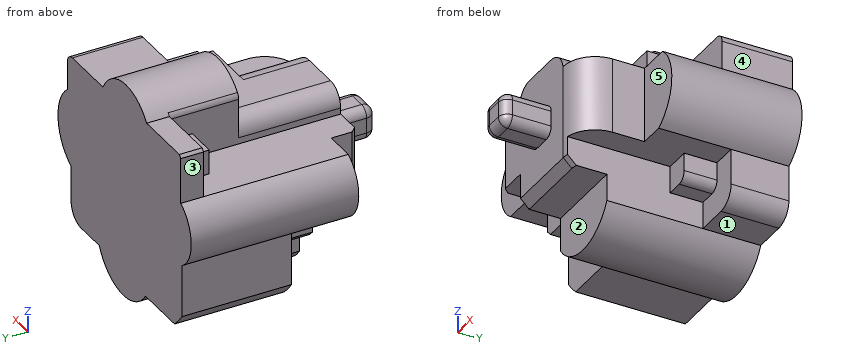
```python
from build123d import *

# Parameters (mm, degrees)
F0_W         = 19.224062562
F0_H         = 18.6825376004
F1_DEPTH     = 134.874
F2_DEPTH     = 108.204
F0_W_2       = 18.3131638914
F0_H_2       = 18.7943680212
F3_DEPTH     = 83.058
F0_W_3       = 17.1565823257
F0_H_3       = 13.6970020831
F4_DEPTH     = 25.4
F0_W_4       = 17.9688669741
F0_H_4       = 10.4478634894
F5_DEPTH     = 71.374
F0_W_5       = 14.1782090068
F0_H_5       = 15.0508098304
F6_DEPTH     = 50.546
F7_DEPTH     = 72.644
F8_DEPTH     = 85.852
F9_DEPTH     = 51.308
F10_DEPTH    = 93.472
F11_DEPTH    = 61.214
F12_DEPTH    = 32.258
F13_DEPTH    = 39.37
F14_DEPTH    = 12.7
F15_R        = 5.08
F16_R        = 10.16
F17_R        = 5.08
F18_T1_DEPTH = 68.0767879487
F19_R        = 10.16
F20_SIZE     = 3.0226
F21_R        = 17.78
F22_SIZE     = 4.8203104
F23_R        = 5.08
F24_R        = 5.08
F25_R        = 5.08
F26_R        = 5.08
F27_R        = 5.08


# Not quite as in the source:
# - a fillet or chamfer that OpenCascade refuses, or shapes differently, is made with other operations: its cross-section is extruded or revolved along the edge and cut away or added


with BuildPart() as f1:
    # F0 (on Front) → F1 (new body)
    with BuildSketch(Plane.XZ):
        Rectangle(F0_W, F0_H)
    extrude(amount=F1_DEPTH)

    # F0 (on Front) → F2 (join)
    with BuildSketch(Plane.XZ):
        Polygon((-21.2547723204, -33.8216274977), (25.389727205, -33.8216274977), (25.389727205, -18.7708176672), (39.5679362118, -18.7708176672), (39.5679362118, 23.3737640083), (21.5990692377, 23.3737640083), (21.5990692377, 33.8216274977), (-22.4113538861, 33.8216274977), (-22.4113538861, 20.1246254146), (-39.5679362118, 20.1246254146), (-39.5679362118, -15.0272594765), (-21.2547723204, -15.0272594765), align=None)
        Rectangle(F0_W, F0_H, mode=Mode.SUBTRACT)
    extrude(amount=F2_DEPTH)

    # F0 (on Front) → F3 (join)
    with BuildSketch(Plane.XZ):
        with Locations((-30.4113542661, -24.4244434871)):
            Rectangle(F0_W_2, F0_H_2)
    extrude(amount=F3_DEPTH)

    # F0 (on Front) → F4 (join)
    with BuildSketch(Plane.XZ):
        with Locations((-30.989645049, 26.9731264561)):
            Rectangle(F0_W_3, F0_H_3)
    extrude(amount=F4_DEPTH)

    # F0 (on Front) → F5 (join)
    with BuildSketch(Plane.XZ):
        with Locations((30.5835027248, 28.597695753)):
            Rectangle(F0_W_4, F0_H_4)
    extrude(amount=F5_DEPTH)

    # F0 (on Front) → F6 (join)
    with BuildSketch(Plane.XZ):
        with Locations((32.4788317084, -26.2962225825)):
            Rectangle(F0_W_5, F0_H_5)
    extrude(amount=F6_DEPTH)

    # F0 (on Front) → F7 (join)
    with BuildSketch(Plane.XZ):
        with BuildLine():
            Line((39.5679362118, 23.3737640083), (39.5679362118, -18.7708176672))
            Line((39.5679362118, -18.7708176672), (53.7461452186, -18.7708176672))
            ThreePointArc((53.7461452186, -18.7708176672), (66.8748667644, 1.2910953871), (57.5368031859, 23.3737640083))
            Line((57.5368031859, 23.3737640083), (39.5679362118, 23.3737640083))
        make_face()
    extrude(amount=F7_DEPTH)

    # F0 (on Front) → F8 (join)
    with BuildSketch(Plane.XZ):
        with BuildLine():
            Line((25.389727205, -48.8724373281), (25.389727205, -33.8216274977))
            Line((25.389727205, -33.8216274977), (-21.2547723204, -33.8216274977))
            Line((-21.2547723204, -33.8216274977), (-21.2547723204, -52.6159955189))
            ThreePointArc((-21.2547723204, -52.6159955189), (3.1426231279, -64.1404640217), (25.389727205, -48.8724373281))
        make_face()
    extrude(amount=F8_DEPTH)

    # F0 (on Front) → F9 (join)
    with BuildSketch(Plane.XZ):
        with BuildLine():
            Line((-22.4113538861, 33.8216274977), (21.5990692377, 33.8216274977))
            Line((21.5990692377, 33.8216274977), (21.5990692377, 44.2694909871))
            ThreePointArc((21.5990692377, 44.2694909871), (0.4961178031, 58.1154072117), (-22.4113538861, 47.5186295807))
            Line((-22.4113538861, 47.5186295807), (-22.4113538861, 33.8216274977))
        make_face()
    extrude(amount=F9_DEPTH)

    # F0 (on Front) → F10 (join)
    with BuildSketch(Plane.XZ):
        with BuildLine():
            Line((-57.8811001033, -15.0272594765), (-39.5679362118, -15.0272594765))
            Line((-39.5679362118, -15.0272594765), (-39.5679362118, 20.1246254146))
            Line((-39.5679362118, 20.1246254146), (-56.7245185375, 20.1246254146))
            ThreePointArc((-56.7245185375, 20.1246254146), (-67.2856136398, 2.8771412434), (-57.8811001033, -15.0272594765))
        make_face()
    extrude(amount=F10_DEPTH)

    # F0 (on Front) → F11 (join)
    with BuildSketch(Plane.XZ):
        with BuildLine():
            Line((-21.2547723204, -52.6159955189), (-21.2547723204, -33.8216274977))
            Line((-21.2547723204, -33.8216274977), (-39.5679362118, -33.8216274977))
            Line((-39.5679362118, -33.8216274977), (-39.5679362118, -15.0272594765))
            Line((-39.5679362118, -15.0272594765), (-57.8811001033, -15.0272594765))
            Line((-57.8811001033, -15.0272594765), (-57.8811001033, -44.4008079084))
            ThreePointArc((-57.8811001033, -44.4008079084), (-54.3606128257, -48.647479537), (-50.5293034549, -52.6159955189))
            Line((-50.5293034549, -52.6159955189), (-21.2547723204, -52.6159955189))
        make_face()
    extrude(amount=F11_DEPTH)

    # F0 (on Front) → F12 (join)
    with BuildSketch(Plane.XZ):
        Polygon((39.5679362118, -18.7708176672), (39.5679362118, -33.8216274977), (25.389727205, -33.8216274977), (25.389727205, -48.8724373281), (53.7461452186, -48.8724373281), (53.7461452186, -18.7708176672), align=None)
    extrude(amount=F12_DEPTH)

    # F0 (on Front) → F13 (join)
    with BuildSketch(Plane.XZ):
        Polygon((39.5679362118, 33.8216274977), (39.5679362118, 23.3737640083), (57.5368031859, 23.3737640083), (57.5368031859, 44.2694909871), (21.5990692377, 44.2694909871), (21.5990692377, 33.8216274977), align=None)
    extrude(amount=F13_DEPTH)

    # F0 (on Front) → F14 (join)
    with BuildSketch(Plane.XZ):
        with BuildLine():
            Line((-56.7245185375, 20.1246254146), (-39.5679362118, 20.1246254146))
            Line((-39.5679362118, 20.1246254146), (-39.5679362118, 33.8216274977))
            Line((-39.5679362118, 33.8216274977), (-22.4113538861, 33.8216274977))
            Line((-22.4113538861, 33.8216274977), (-22.4113538861, 47.5186295807))
            Line((-22.4113538861, 47.5186295807), (-55.3500978757, 47.5186295807))
            ThreePointArc((-55.3500978757, 47.5186295807), (-56.0433767246, 46.6989659134), (-56.7245185375, 45.8691888828))
            Line((-56.7245185375, 45.8691888828), (-56.7245185375, 20.1246254146))
        make_face()
    extrude(amount=F14_DEPTH)

    # F15
    f15_edges = [f1.edges().sort_by_distance(p)[0] for p in [
        (57.536803, -19.685, 44.269491),
    ]]
    fillet(f15_edges, radius=F15_R)

    # F16
    f16_edges = [f1.edges().sort_by_distance(p)[0] for p in [
        (53.746145, -16.129, -48.872437),
    ]]
    fillet(f16_edges, radius=F16_R)

    # F17
    f17_edges = [f1.edges().sort_by_distance(p)[0] for p in [
        (39.567936, -41.402, -33.821627),
    ]]
    fillet(f17_edges, radius=F17_R)

    # F18: fillet of radius 12.7 on 1 edges, made by hand

    # F18_s2 → F18_t1 (cut)
    with BuildSketch(Plane.XZ.offset(71.374)):
        with BuildLine():
            ThreePointArc((21.5990692377, 23.3737640083), (17.2455325804, 30.8656547371), (9.1003540582, 33.8216274977))
            Line((9.1003540582, 33.8216274977), (21.5990692377, 33.8216274977))
            Line((21.5990692377, 33.8216274977), (21.5990692377, 23.3737640083))
        make_face()
    extrude(amount=F18_T1_DEPTH, mode=Mode.SUBTRACT)

    # F19
    f19_edges = [f1.edges().sort_by_distance(p)[0] for p in [
        (-22.411354, -79.756, 33.821627),
    ]]
    fillet(f19_edges, radius=F19_R)

    # F20
    f20_edges = [f1.edges().sort_by_distance(p)[0] for p in [
        (-39.567936, -72.136, -33.821627),
        (-39.567936, -108.204, 2.548683),
    ]]
    chamfer(f20_edges, length=F20_SIZE)

    # F21
    f21_edges = [f1.edges().sort_by_distance(p)[0] for p in [
        (39.567936, -108.204, 2.301473),
    ]]
    fillet(f21_edges, radius=F21_R)

    # F22
    f22_edges = [f1.edges().sort_by_distance(p)[0] for p in [
        (0.266582, -108.204, -33.821627),
        (23.59824, -108.1116, -33.821627),
    ]]
    chamfer(f22_edges, length=F22_SIZE)

    # F23
    f23_edges = [f1.edges().sort_by_distance(p)[0] for p in [
        (0, -134.874, -9.341269),
    ]]
    fillet(f23_edges, radius=F23_R)

    # F24
    f24_edges = [f1.edges().sort_by_distance(p)[0] for p in [
        (-9.612031, -134.874, 2.54),
    ]]
    fillet(f24_edges, radius=F24_R)

    # F25
    f25_edges = [f1.edges().sort_by_distance(p)[0] for p in [
        (2.54, -134.874, 9.341269),
    ]]
    fillet(f25_edges, radius=F25_R)

    # F26
    f26_edges = [f1.edges().sort_by_distance(p)[0] for p in [
        (9.612031, -134.874, 0),
    ]]
    fillet(f26_edges, radius=F26_R)

    # F27
    f27_edges = [f1.edges().sort_by_distance(p)[0] for p in [
        (-22.411354, -32.004, 47.51863),
    ]]
    fillet(f27_edges, radius=F27_R)


solid = f1.part
```
Here's how the part is built. I have some questions about the finished solid (model axes, mm). Face numbers are marked on the shaded views. A direction names the side the tool comes from. Coordinates: 2 decimals unless noted, no trailing zeros. Loops run counter-clockwise (first coordinate to the right, second up) from the corner with the lowest first, then second, coordinate; pieces in that order, holes last. Notation, with made-up numbers: (10.5, 81) - (35.5, 81) arc R23 ccw to (35.5, 117) - close; hole circle Ø11 at (87, 2). An arc over 180 degrees is marked (long way). Return JSON: item names as keys, results as strings. Group by question number.
Item 1: If we section it at B-B on y = -37: Write out the boundary of the cut face in (x, z), and give its area (3 significant figures).
Item 2: I need wall thicknesses on line 1 (X direction, y = -16, z = 38); line 2 (X direction, y = -92, z = -20); line 3 (Y direction, x = -4, z = 11.5). Which ranges of each line are inside material? Lowest first, please. Write a range as from..to.
Item 3: If we section it at A-A on x = -47: Write out the boundary of the cut face in (y, z), and give its area (3 significant figures).
Item 4: If we section it at D-D on x = -28: Write out the boundary of the cut face in (y, z), and give its area (3 significant figures).
Item 5: On a 3-axis mill with a long thin cutter (end or side, diameter ignored), from which of +Z, -Z, +X, -X, +Y, -Y can I reach the whole of each face in a straight line? I mean the marked faces 1, 2, 3, 4 and 5. Say none if no direction works.
Item 6: Will these pins go through, and if not, where does the flat tip stop? P1, Ø4, axis at x = -29, z = 29.5, coming from the -Y side; P2, Ø2.5, axis at x = 0, y = -123, coming from the +Z side; P3, Ø8.5, axis at x = 42.5, z = -29, coming from the -Y side.
Item 7: If we section it at C-C on z = 14: Write out the boundary of the cut face in (x, y), and give its area (3 significant figures).
Calculated:
{
 "1": {"outline": "(-57.88, -44.4) arc R72.95 ccw to (-50.53, -52.62) - (-21.25, -52.62) arc R27.09 ccw to (25.39, -48.87) - (25.39, -33.82) - (34.49, -33.82) arc R5.08 ccw to (39.57, -28.74) - (39.57, -18.77) - (53.75, -18.77) arc R25.48 ccw to (57.54, 23.37) - (57.54, 39.19) arc R5.08 ccw to (52.46, 44.27) - (21.6, 44.27) arc R25.99 ccw to (-21.2, 49.06) arc R5.08 ccw to (-22.41, 45.76) - (-22.41, 20.12) - (-56.72, 20.12) arc R20.47 ccw to (-57.88, -15.03) - close", "area": "10,700 mm^2"},
 "2": {"line 1": "x = -22.41..57.54", "line 2": "x = -21.25..25.39", "line 3": "y = -108.2..0"},
 "3": {"outline": "(-93.47, -15.03) - (-61.21, -15.03) - (-61.21, -52.62) - (0, -52.62) - (0, 47.52) - (-12.7, 47.52) - (-12.7, 20.12) - (-93.47, 20.12) - close", "area": "5,930 mm^2"},
 "4": {"outline": "(-108.2, -15.03) - (-83.06, -15.03) - (-83.06, -33.82) - (-61.21, -33.82) - (-61.21, -52.62) - (0, -52.62) - (0, 47.52) - (-12.7, 47.52) - (-12.7, 33.82) - (-25.4, 33.82) - (-25.4, 20.12) - (-108.2, 20.12) - close", "area": "7,040 mm^2"},
 "5": {"face 1": "-Z, +X, +Y, -Y", "face 2": "-Z, +X, -X, -Y", "face 3": "+Z, -X, +Y, -Y", "face 4": "+Z, +X, +Y, -Y", "face 5": "+Z, -Z, +X, -Y"},
 "6": {"P1": "stops at y = -25.4", "P2": "stops at z = 9.34", "P3": "stops at y = -50.55"},
 "7": {"outline": "(-63.56, -93.47) - (-39.57, -93.47) - (-39.57, -105.18) - (-36.55, -108.2) - (21.79, -108.2) arc R17.78 ccw to (39.57, -90.42) - (39.57, -72.64) - (64.75, -72.64) - (64.75, 0) - (-63.56, 0) - close", "area": "12,600 mm^2"}
}
